The listing builds one solid part. Answer for the finished solid, in the listing's coordinates (mm). Face numbers are marked on the shaded views. Round coordinates to 2 decimals unless told otherwise and drop trailing zeros. Loops run counter-clockwise (first coordinate to the right, second up) from the corner with the lowest first, then second, coordinate; pieces in that order, holes last. Notation, with made-up numbers: M 46.5,73.25 L 68.5,73.25 A16 cw 68.5,94.25 Z; hole C 56.5,-27.75 d2. An arc over 180 degrees is marked long. Put each result on its own line as item: value. Start each with the question number.
(1) Section D-D, the plane z = -3.25 is taken. Determine the outline of the cut face in (x, y), then the cut area to 3 significant figures.
(2) Straight lines are drawn through the part: line 1 (X direction, y = 0.35, z = 0); line 2 (X direction, y = 1.95, z = 0); line 3 (Y direction, x = -7.5, z = -3.5). For each, find the intervals that lie inside material, in ascending order.
(3) Section A-A, the plane z = 0 is taken. Determine the outline of the cut face in (x, y).
(4) Determine the mould class of the marked faces 1, 2 and 3 for opening direction Z: released by +Z, released by -Z, zero draft, split by the parting line, or undercut.
(5) A flat-ended cylindrical pin translates along its axis: P1, Ø1, axis at x = -7.5, z = 3.5, coming from the +Y side. Find the tip coordinate at first contact, or state that the pin passes through.
(6) Section B-B, the plane x = -6 is taken. Determine the outline of the cut face in (y, z), then the cut area to 3 significant figures.
(7) Section C-C, the plane y = 0.7 is taken. Determine the outline of the cut face in (x, z), then the cut area to 3 significant figures.
```python
from build123d import *

# Parameters (mm, degrees)
SKETCH_1_W          = 22
SKETCH_1_H          = 9.5
EXTRUDE_1_DEPTH     = 2.5
SKETCH_2_R          = 4
CUT_EXTRUDE_1_DEPTH = 13.983162173
SKETCH_3_R          = 4
CUT_EXTRUDE_2_DEPTH = 1
SKETCH_4_R          = 3
CUT_EXTRUDE_3_DEPTH = 13.631805097
CHAMFER_1_SIZE      = 2


with BuildPart() as part:
    # 草图1 → 凸台-拉伸1 (new, symmetric)
    with BuildSketch(Plane(origin=(0, 0, 0), x_dir=(1, 0, 0), z_dir=(0, 1, 0))):
        Rectangle(SKETCH_1_W, SKETCH_1_H)
    extrude(amount=EXTRUDE_1_DEPTH, both=True)

    # 草图2 → 切除-拉伸1 (cut, through all)
    with BuildSketch(Plane(origin=(0, 2.5, 0), x_dir=(1, 0, 0), z_dir=(0, 1, 0))):
        with Locations(Location((6, 0, 0), (0, 0, 270))):
            Circle(SKETCH_2_R)
    extrude(amount=-CUT_EXTRUDE_1_DEPTH, mode=Mode.SUBTRACT)

    # 草图3 → 切除-拉伸2 (cut)
    with BuildSketch(Plane(origin=(0, 2.5, 0), x_dir=(1, 0, 0), z_dir=(0, 1, 0))):
        with Locations(Location((-6, 0, 0), (0, 0, 270))):
            Circle(SKETCH_3_R)
    extrude(amount=-CUT_EXTRUDE_2_DEPTH, mode=Mode.SUBTRACT)

    # 草图4 → 切除-拉伸3 (cut, through all)
    with BuildSketch(Plane(origin=(0, 1.5, 0), x_dir=(1, 0, 0), z_dir=(0, 1, 0))):
        with Locations(Location((-6, 0, 0), (0, 0, 270))):
            Circle(SKETCH_4_R)
    extrude(amount=-CUT_EXTRUDE_3_DEPTH, mode=Mode.SUBTRACT)

    # 倒角1
    chamfer_1_edges = [part.edges().sort_by_distance(p)[0] for p in [
        (-11, 0, -4.75),
        (11, 0, -4.75),
        (11, 0, 4.75),
        (-11, 0, 4.75),
    ]]
    chamfer(chamfer_1_edges, length=CHAMFER_1_SIZE)


solid = part.part
```
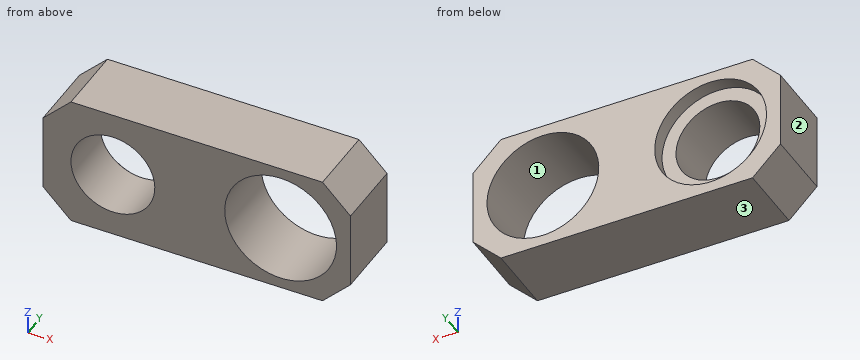
Recorded:
1. outline: M -10.5,-2.5 L 3.67,-2.5 L 3.67,2.5 L -3.67,2.5 L -3.67,1.5 L -8.33,1.5 L -8.33,2.5 L -10.5,2.5 Z; M 8.33,-2.5 L 10.5,-2.5 L 10.5,2.5 L 8.33,2.5 Z
1. area: 77.0 mm²
2. line 1: x = -11 to -9, -3 to 2, 10 to 11
2. line 2: x = -11 to -10, -2 to 2, 10 to 11
2. line 3: y = -2.5 to 1.5
3. outline: M -11,-2.5 L -9,-2.5 L -9,1.5 L -10,1.5 L -10,2.5 L -11,2.5 Z; M -3,-2.5 L 2,-2.5 L 2,2.5 L -2,2.5 L -2,1.5 L -3,1.5 Z; M 10,-2.5 L 11,-2.5 L 11,2.5 L 10,2.5 Z
4. face 1: undercut
4. face 2: zero draft
4. face 3: released by -Z
5. P1: stops at y = 2.5
6. outline: M -2.5,-4.75 L 2.5,-4.75 L 2.5,-4 L 1.5,-4 L 1.5,-3 L -2.5,-3 Z; M -2.5,3 L 1.5,3 L 1.5,4 L 2.5,4 L 2.5,4.75 L -2.5,4.75 Z
6. area: 15.5 mm²
7. outline: M -11,-2.75 L -9,-4.75 L 9,-4.75 L 11,-2.75 L 11,2.75 L 9,4.75 L -9,4.75 L -11,2.75 Z; hole C -6,0 d6; hole C 6,0 d8
7. area: 122 mm²
